The listing builds one solid part. Answer for the finished solid, in the listing's coordinates (mm). A direction names the side the tool comes from. Round coordinates to 2 decimals unless told otherwise and drop trailing zeros. Loops run counter-clockwise (first coordinate to the right, second up) from the corner with the lowest first, then second, coordinate; pieces in that order, holes last. Notation, with made-up numbers: M 50.5,-32.5 L 72.5,-32.5 A15 cw 72.5,-15.5 Z; hole C -31.5,19 d11. An arc over 180 degrees is marked long. Put each result on its own line as item: value. Start each with the question number.
(1) Section A-A, the plane z = 10.16 is taken. Determine the outline of the cut face in (x, y).
(2) Section B-B, the plane x = 21 is taken. Determine the outline of the cut face in (y, z).
(3) Section D-D, the plane y = -14.5 is taken. Determine the outline of the cut face in (x, z).
(4) Straight lines are drawn through the part: line 1 (X direction, y = -0.25, z = 10.16); line 2 (Y direction, x = 30.5, z = 18.5); line 3 (Z direction, x = 19.5, y = 9.5). For each, find the intervals that lie inside material, in ascending order.
(5) Flat-ended cylindrical pins translate along their axes: P1, Ø4.5, axis at x = 28, z = 13, coming from the +Y side; P2, Ø1.4, axis at x = 3.5, z = 0.5, coming from the -Y side; P3, Ø1, axis at x = 27, z = 0.5, coming from the +Y side; P4, Ø4.5, axis at y = -5.5, z = 14, coming from the +X side. Find the tip coordinate at first contact, or state that the pin passes through.
(6) Which of the six approach directions +Z, -Z, +X, -X, +Y, -Y give full straight-line access (tool end or side, diameter ignored) to faces 1 (the face through (18, -8.89, 1)), 2 (the face through (6, 9.652, 1)), 3 (the face through (19.304, 11, 1)), 4 (the face through (30, 0, 11))?
(7) Determine the mould class of faces 5 (the face through (10.9, -18.3, 19.7)), 6 (the face through (23.876, -5, 1)), 7 (the face through (30, -1.27, 10)), 8 (the face through (12.954, -1, 14)) for opening direction X: released by +X, released by -X, zero draft, split by the parting line, or undercut.
(8) Section C-C, the plane z = 17.25 is taken. Determine the outline of the cut face in (x, y).
```python
from build123d import *

# Parameters (mm, degrees)
BOSS_EXTRUDE1_DEPTH = 1.27
SKETCH4_W           = 8.636
SKETCH4_H           = 1.27
SKETCH4_W_2         = 2.794
BOSS_EXTRUDE2_DEPTH = 20.32
SKETCH5_W           = 2.794
SKETCH5_H           = 1.27
SKETCH5_W_2         = 7.366
BOSS_EXTRUDE3_DEPTH = 7.62
BOSS_EXTRUDE4_DEPTH = 1.27
SKETCH7_R           = 1.524
CUT_EXTRUDE1_DEPTH  = 49.663543079


with BuildPart() as part:
    # Sketch1 → Boss-Extrude1 (new body)
    with BuildSketch(Plane.XY):
        with BuildLine():
            Line((0, 0), (0, 9.652))
            Line((0, 9.652), (11.684, 9.652))
            Line((11.684, 9.652), (11.684, 13.208))
            ThreePointArc((11.684, 13.208), (15.494, 17.018), (19.304, 13.208))
            Line((19.304, 13.208), (19.304, 9.652))
            Line((19.304, 9.652), (32.639, 9.652))
            Line((32.639, 9.652), (32.639, 13.208))
            ThreePointArc((32.639, 13.208), (36.449, 17.018), (40.259, 13.208))
            Line((40.259, 13.208), (40.259, 9.652))
            Line((40.259, 9.652), (40.259, 0))
            Line((40.259, 0), (23.876, 0))
            Line((23.876, 0), (23.876, -8.89))
            Line((23.876, -8.89), (12.954, -8.89))
            Line((12.954, -8.89), (12.954, 0))
            Line((12.954, 0), (0, 0))
        make_face()
    extrude(amount=BOSS_EXTRUDE1_DEPTH)

    # Sketch4 → Boss-Extrude2 (add)
    with BuildSketch(Plane.XY):
        with Locations((28.194, -0.635)):
            Rectangle(SKETCH4_W, SKETCH4_H)
        with Locations((11.557, -0.635)):
            Rectangle(SKETCH4_W_2, SKETCH4_H)
    extrude(amount=BOSS_EXTRUDE2_DEPTH)

    # Sketch5 → Boss-Extrude3 (add)
    with BuildSketch(Plane.XZ.offset(1.27)):
        with Locations((11.557, 19.685)):
            Rectangle(SKETCH5_W, SKETCH5_H)
        with Locations((27.559, 19.685)):
            Rectangle(SKETCH5_W_2, SKETCH5_H)
    extrude(amount=BOSS_EXTRUDE3_DEPTH)

    # Sketch6 → Boss-Extrude4 (add)
    with BuildSketch(Plane(origin=(0, 0, 19.05), x_dir=(-1, 0, 0), z_dir=(0, 0, -1))):
        with BuildLine():
            Line((-10.16, -8.89), (-31.242, -8.89))
            Line((-31.242, -8.89), (-31.242, -16.51))
            ThreePointArc((-31.242, -16.51), (-30.498051224, -18.306051224), (-28.702, -19.05))
            Line((-28.702, -19.05), (-12.7, -19.05))
            ThreePointArc((-12.7, -19.05), (-10.903948776, -18.306051224), (-10.16, -16.51))
            Line((-10.16, -16.51), (-10.16, -8.89))
        make_face()
    extrude(amount=-BOSS_EXTRUDE4_DEPTH)

    # Sketch7 → Cut-Extrude1 (cut, through all)
    with BuildSketch(Plane.XZ.offset(1.27)):
        with Locations(Location((28.194, 10.16, 0), (0, 0, 270))):
            Circle(SKETCH7_R)
    extrude(amount=-CUT_EXTRUDE1_DEPTH, mode=Mode.SUBTRACT)


solid = part.part
```
Recorded:
1. outline: M 10.16,-1.27 L 12.95,-1.27 L 12.95,0 L 10.16,0 Z; M 23.88,-1.27 L 26.67,-1.27 L 26.67,0 L 23.88,0 Z; M 29.72,-1.27 L 32.51,-1.27 L 32.51,0 L 29.72,0 Z
2. outline: M -19.05,19.05 L -8.89,19.05 L -8.89,20.32 L -19.05,20.32 Z; M -8.89,0 L 9.65,0 L 9.65,1.27 L -8.89,1.27 Z
3. outline: M 10.16,19.05 L 31.24,19.05 L 31.24,20.32 L 10.16,20.32 Z
4. line 1: x = 10.16 to 12.95, 23.88 to 26.67, 29.72 to 32.51
4. line 2: y = -1.27 to 0
4. line 3: z = 0 to 1.27
5. P1: stops at y = 0
5. P2: stops at y = 0
5. P3: stops at y = 9.65
5. P4: passes through
6. face 1: -Z, +X, -X, -Y
6. face 2: +Z, -Z, -X, +Y
6. face 3: +Z, -Z, +Y
6. face 4: +Z, +X, -X, +Y
7. face 5: released by -X
7. face 6: released by +X
7. face 7: zero draft
7. face 8: undercut
8. outline: M 10.16,-1.27 L 12.95,-1.27 L 12.95,0 L 10.16,0 Z; M 23.88,-1.27 L 32.51,-1.27 L 32.51,0 L 23.88,0 Z
